Could you check a few things on this model? Use its own coordinates, in mm. Round coordinates to 2 decimals unless told otherwise and drop trailing zeros. Loops run counter-clockwise (first coordinate to the right, second up) from the corner with the lowest first, then second, coordinate; pieces in that order, holes last. Notation, with made-up numbers: (51, 32) -> (109, 32) arc R6 cw to (109, 37) -> close; hole circle Ø3 at (43, 69.25). An arc over 180 degrees is marked (long way). Put each result on its own line as item: value. Start each with the question number.
1. If we mould it in two halves opening along X, with no side actions, what happens to faces 1 (the cylindrical face through (-6.73, 0.15, 5.65)), 2 (the cylindrical face through (30.522, 4.753, 5.647)), 3 (the cylindrical face through (4.028, 1.268, 5.635)), 4 (the cylindrical face through (12.88, 6.46, 0.25))? For each: pulls with the +X half, pulls with the -X half, needs draft (parallel to the pull), parting line crosses it, or undercut.
2. Imagine slicing it at A-A, the plane z = 4.25. Please give me the cut outline in (x, y), and give its area (3 significant figures).
3. I'm going to push flat-ended pins straight in: P1, Ø3, axis at x = 1, y = -1.5, coming from the +Z side; P2, Ø1.5, axis at y = -4.5, z = 5, coming from the +X side; P3, Ø2, axis at y = 3, z = 1.5, coming from the +X side. Where does each tip first touch, or does it pass through?
4. I need wall thicknesses on line 1 (Y direction, x = 0, z = 8); line 2 (X direction, y = 3, z = 3); line 3 (X direction, y = -3.25, z = 1.5). Which ranges of each line are inside material? Lowest first, please. Write a range as [from, to].
```python
from build123d import *

# Parameters (mm, degrees)
SKETCH1_R           = 6.731
SKETCH1_R_2         = 4.22275
BOSS_EXTRUDE1_DEPTH = 11.43
FRONT_FILLET_R      = 7.62
SIDE_FILLET_R       = 0.889


with BuildPart() as part:
    # Sketch1 → Boss-Extrude1 (new body)
    # profile 1 of 2: a face of its own
    with BuildSketch(Plane.XY):
        with BuildLine():
            Line((33.02, 6.731), (0, 6.731))
            ThreePointArc((0, 6.731), (4.759535744, 4.759535744), (6.731, 0))
            ThreePointArc((6.731, 0), (4.759535744, -4.759535744), (0, -6.731))
            Line((0, -6.731), (33.02, -6.731))
            Line((33.02, -6.731), (33.02, 6.731))
        make_face()
    # profile 2 of 2: a face of its own
    with BuildSketch(Plane.XY):
        Circle(SKETCH1_R)
        Circle(SKETCH1_R_2, mode=Mode.SUBTRACT)
    extrude(amount=BOSS_EXTRUDE1_DEPTH)

    # Front Fillet
    # the kernel refuses this fillet: 7.62 mm, written as the material it takes off along each edge
    with BuildSketch(Plane(origin=(33.02, -6.731, -19.05), x_dir=(-1, 0, 0), z_dir=(0, 0, 1)), Plane(origin=(33.02, 6.731, -19.05), x_dir=(0, -1, 0), z_dir=(0, 0, 1))) as front_fillet_piece_1:
        with BuildLine():
            CenterArc((FRONT_FILLET_R, -FRONT_FILLET_R), FRONT_FILLET_R, 90, 90)
            Line((0, -FRONT_FILLET_R), (0, 0))
            Line((0, 0), (FRONT_FILLET_R, 0))
        make_face()
    extrude(amount=49.53, mode=Mode.SUBTRACT)

    # Side Fillet
    side_fillet_edges = [part.edges().sort_by_distance(p)[0] for p in [
        (-6.731, 0, 11.43),
        (12.7, -6.731, 11.43),
        (30.464100117, 4.80479399, 0),
        (30.464100117, -4.80479399, 0),
        (30.464100117, 4.80479399, 11.43),
        (30.464100117, -4.80479399, 11.43),
        (12.7, 6.731, 11.43),
        (12.7, -6.731, 0),
        (-6.731, 0, 0),
        (12.7, 6.731, 0),
    ]]
    fillet(side_fillet_edges, radius=SIDE_FILLET_R)


solid = part.part
```
Entries:
1. face 1: pulls with the -X half
1. face 2: pulls with the +X half
1. face 3: undercut
1. face 4: needs draft
2. outline: (0, -6.73) -> (25.4, -6.73) arc R7.62 ccw to (32.97, 0) arc R7.62 ccw to (25.4, 6.73) -> (0, 6.73) arc R6.73 ccw to start; hole circle Ø8.45 at (0, 0)
2. area: 435 mm^2
3. P1: through
3. P2: x = 31.45
3. P3: x = 32.45
4. line 1: [-6.73, -4.22], [4.22, 6.73]
4. line 2: [-6.03, -2.97], [2.97, 31.95]
4. line 3: [-5.89, -2.7], [2.7, 31.8]
